Verification items for the finished model (mm, model axes). Coordinates: 2 decimals unless noted, no trailing zeros. Order: outer loops, then holes, each group sorted by start corner. A loop starts at its lowest first (then second) coordinate and runs counter-clockwise, first axis right, second up. Notation, with made-up numbers: (16, -19) -> (41, -19) arc R13 ccw to (41, -8) -> close; hole circle Ø6 at (-3, -8). An arc over 180 degrees is marked (long way). Write each question's results on one line, items separated by ' | '. Start each with the question number.
(1) Go/stop test with flat-tipped pins: pin 1 (6 mm diameter, centred on x = 3.5, y = -3, fed in from -Z); pin 2 (5 mm diameter, centred on y = -3, z = 2, fed in from +X); pin 3 (4 mm diameter, centred on x = 2.5, z = 2.5, fed in from -Y); pin 4 (1 mm diameter, centred on x = -1, z = 6, fed in from -Y). Record where each tip stops, or that it passes through.
(2) Cross-section at A-A on z = 8.25. Enter the section's corners in (x, y), and give its area (3 significant figures).
(3) Draft check along Y on faces 1 (the flat face through (3, -1, 2)), 2 (the cylindrical face through (-1.4, 0.06, 6.06)), 3 (the cylindrical face through (-2.262, -1.734, 5.451)). Enter one of: +Y half, -Y half, draft (parallel to the pull), parting line (faces both ways), or undercut.
(4) Thickness scan on probe 1 along Y at (x, z) = (0, 4.7); probe 2 along Z at (x, y) = (2, -2.5); probe 3 along Y at (x, z) = (1, 6.5). Record the ranges inside material, lowest first. Write a range as [from, to].
```python
from build123d import *

# Parameters (mm, degrees)
F0_R     = 6
F1_DEPTH = 2
F2_SIZE2 = 2.5980762114
F2_SIZE  = 1.5
F4_R     = 2.85
F4_R_2   = 1.4
F5_DEPTH = 7
F6_R     = 1.2


# Not quite as in the source:
# - a fillet or chamfer that OpenCascade refuses, or shapes differently, is made with other operations: its cross-section is extruded or revolved along the edge and cut away or added


with BuildPart() as f1:
    # F0 (on Top) → F1 (new body)
    with BuildSketch(Plane.XY):
        Circle(F0_R)
    extrude(amount=F1_DEPTH)

    # F2
    f2_edges = [f1.edges().sort_by_distance(p)[0] for p in [
        (-6, 0, 0),
    ]]
    f2_side = f1.faces().sort_by_distance((-6, 0, 1))[0]
    chamfer(f2_edges, length=F2_SIZE, length2=F2_SIZE2, reference=f2_side)

    # F3: fillet of radius 1 on 2 edges, made by hand

    # F3_s1 → F3_t2 (revolve, cut)
    with BuildSketch(Plane.XZ):
        with BuildLine():
            ThreePointArc((3.6339745962, 0.1339745962), (3.3927936413, 0.0340741737), (3.1339745962, 0))
            Line((3.1339745962, 0), (3.4019237886, 0))
            Line((3.4019237886, 0), (3.6339745962, 0.1339745962))
        make_face()
    revolve(axis=Axis((0, 0, 0), (0, 0, 1)), mode=Mode.SUBTRACT)

    # F3_s3 → F3_t4 (revolve, cut)
    with BuildSketch(Plane.XZ):
        with BuildLine():
            ThreePointArc((6, 2), (5.8486778537, 1.5452494356), (5.5031382462, 1.2131367327))
            Line((5.5031382462, 1.2131367327), (6, 1.5))
            Line((6, 1.5), (6, 2))
        make_face()
    revolve(axis=Axis((0, 0, 1.5), (0, 0, 1)), mode=Mode.SUBTRACT)

    # F4 (on face) → F5 (join)
    with BuildSketch(Plane.XY.offset(2)):
        Circle(F4_R)
        Circle(F4_R_2, mode=Mode.SUBTRACT)
    extrude(amount=F5_DEPTH)

    # F6
    f6_edges = [f1.edges().sort_by_distance(p)[0] for p in [
        (-1.4, 0, 2),
    ]]
    fillet(f6_edges, radius=F6_R)


solid = f1.part
```
Results are:
1) pin 1: stops at z = 0 | pin 2: stops at x = 5.98 | pin 3: stops at y = -5.97 | pin 4: stops at y = -2.81
2) outline: circle Ø5.7 at (0, 0); hole circle Ø2.8 at (0, 0) | area: 19.4 mm2
3) face 1: draft | face 2: undercut | face 3: parting line
4) probe 1: y = [-2.85, -1.4], [1.4, 2.85] | probe 2: z = [0, 2] | probe 3: y = [-2.67, -0.98], [0.98, 2.67]
